Autodesk Inventor part; units mm, degrees
ref_plane "YZ Plane" through (0, 0, 0) normal (1, 0, 0) x (0, 1, 0)
ref_plane "XZ Plane" through (0, 0, 0) normal (0, 1, 0) x (-1, 0, 0)
ref_plane "XY Plane" through (0, 0, 0) normal (0, 0, 1) x (1, 0, 0)
sketch "Sketch1" plane through (0, 0, 0) normal (0, 0, 1) x (1, 0, 0)
  line L0 (0, 0) -> (-5, 0)
  line L1 (-5, 5) -> (-5, 50)
  line L2 (-5, 50) -> (0, 50)
  line L3 (0, 50) -> (0, 0)
  line L4 (0, 0) -> (-50, 0)
  line L5 (-50, 0) -> (-50, 5)
  line L6 (-50, 5) -> (-5, 5)
  line L7 (0, 5) -> (0, 0)
  dimension "d0" = 5
  dimension "d1" = 50
  dimension "d2" = 50
  dimension "d3" = 5
extrude "Extrusion1" add sketch "Sketch1" along normal blind 50
sketch "Sketch3" plane through (-50, 5, 0) normal (0, 1, 0) x (1, 0, 0)
  circle A0 centre (22.5, -25) radius 14.5
  line L0 (45, 0) -> (0, 0)
  line L1 (0, 0) -> (0, -50)
  line L2 (45, -50) -> (0, -50)
  line L3 (45, 0) -> (45, -50)
  line L4 (22.5, -25) -> (0, -25)
  line L5 (22.5, -25) -> (22.5, 0)
  line L6 (45, 0) -> (0, 0)
  circle A1 centre (35.935, -38.435) radius 2.75
  circle A2 centre (9.065, -38.435) radius 2.75
  circle A3 centre (22.5, -44) radius 2.75
  circle A4 centre (35.935, -11.565) radius 2.75
  circle A5 centre (9.065, -11.565) radius 2.75
  circle A6 centre (22.5, -6) radius 2.75
  point P0 (50, 0)
  dimension "d44" = 29
  dimension "d45" = 45
  dimension "d46" = 22.5
  dimension "d47" = 25
  dimension "d48" = 5.5
  dimension "d49" = 13.435
  dimension "d50" = 13.435
  dimension "d51" = 5.5
  dimension "d52" = 13.435
  dimension "d53" = 13.435
  dimension "d54" = 5.5
  dimension "d55" = 19
  dimension "d56" = 0
extrude "Extrusion2" cut sketch "Sketch3" against normal blind 20 contours A0 L4 L5 | L5 L4 A0 | A6 L5 | L5 A6 | A1 | A2 | A3 | A4 | A5
sketch "Sketch4" plane through (-5, 5, 0) normal (-1, 0, 0) x (0, 0, 1)
  circle A0 centre (17.5, 30) radius 2.75
  line L0 (0, 45) -> (0, 0)
  line L1 (0, 45) -> (50, 45)
  circle A1 centre (32.5, 30) radius 2.75
  point P0 (0, -5)
  dimension "d59" = 5.5
  dimension "d61" = 17.5
  dimension "d64" = 45
  dimension "d65" = 15
  dimension "d68" = 5.5
  dimension "d69" = 15
  dimension "d70" = 15
  dimension "d71" = 50
extrude "Extrusion3" cut sketch "Sketch4" against normal blind 20
equation "\"d2\" = d1"
equation "\"d3\" = d0"
equation "\"d46\" = 0.5 * d45"
equation "\"d50\" = d49"
equation "\"d52\" = d49"
equation "\"d53\" = d52"
equation "\"d61\" = -0.5 * d69 + 0.5 * d71"
equation "\"d65\" = -0.5 * d63 + 0.5 * d64"
equation "\"d70\" = d65"
properties part number "LBent_PScrew"
Check sheet for the modelled part. Datum: model origin and axes. Units: mm. A direction names the side the tool comes from. Round coordinates to 2 decimals unless told otherwise and drop trailing zeros. Order: outer loops, then holes, each group sorted by start corner. A loop starts at its lowest first (then second) coordinate and runs counter-clockwise, first axis right, second up.
Q1. Draft check along X on faces 3 (the face through (-13.67, 2.54, 20.64)), 4 (the face through (-38, 5, 36)), 5 (the face through (-29.527, 2.535, 42.141)), 6 (the face through (-50, 2, 25)). Enter one of: pulls with the +X half, pulls with the -X half, needs draft (parallel to the pull), parting line crosses it, or undercut.
Filled sheet:
face 3: undercut
face 4: needs draft
face 5: undercut
face 6: pulls with the -X half
Q2. Cross-section at A-A, the plane y = 35. Enter the section's corners in (x, z), plus the area to 3 significant figures.
Filled sheet:
outline: (-5, 0) - (0, 0) - (0, 14.75) - (-5, 14.75) - close; (-5, 20.25) - (0, 20.25) - (0, 29.75) - (-5, 29.75) - close; (-5, 35.25) - (0, 35.25) - (0, 50) - (-5, 50) - close
area: 195 mm2
Q3. Set-up check for faces 1 (the face through (-13.5, 0, 30.2)), 2 (the face through (-5, 27, 25)): record each of +Z, -Z, +X, -X, +Y, -Y from which the full face is reachable in a straight line by a thin tool's end or side.
Filled sheet:
face 1: +Z, -Z, +X, -X, -Y
face 2: +Z, -Z, -X, +Y
Q4. Scan lines: L1, parallel to Z at x = -27.5, y = 2.6; L2, parallel to Y at x = -23.5, z = 7; L3, parallel to X at y = 6.5, z = 32.5. Record each from-to range of solid material in increasing order.
Filled sheet:
L1: z = 0 to 3.25, 8.75 to 10.5, 39.5 to 41.25, 46.75 to 50
L2: y = 0 to 5
L3: x = -5 to 0
Q5. Cross-section at D-D, the plane z = 31. Enter the section's corners in (x, y), plus the area to 3 significant figures.
Filled sheet:
outline: (-50, 0) - (-40.7, 0) - (-40.7, 5) - (-50, 5) - close; (-14.3, 0) - (0, 0) - (0, 32.7) - (-5, 32.7) - (-5, 5) - (-14.3, 5) - close; (-5, 37.3) - (0, 37.3) - (0, 50) - (-5, 50) - close
area: 320 mm2
Q6. Cross-section at B-B, the plane z = 25. Enter the section's corners in (x, y).
Filled sheet:
outline: (-50, 0) - (-42, 0) - (-42, 5) - (-50, 5) - close; (-13, 0) - (0, 0) - (0, 50) - (-5, 50) - (-5, 5) - (-13, 5) - close
Q7. Cross-section at C-C, the plane x = -27.5. Enter the section's corners in (y, z).
Filled sheet:
outline: (0, 0) - (5, 0) - (5, 3.25) - (0, 3.25) - close; (0, 8.75) - (5, 8.75) - (5, 10.5) - (0, 10.5) - close; (0, 39.5) - (5, 39.5) - (5, 41.25) - (0, 41.25) - close; (0, 46.75) - (5, 46.75) - (5, 50) - (0, 50) - close
Q8. Depth check by flat-ended pin: P1, Ø9, axis at x = -40.935, z = 11.565, coming from the +Y side; P2, Ø2, axis at y = 21.5, z = 41, coming from the -X side. Enter the tip coordinate at first touch or a pass-through.
Filled sheet:
P1: stops at y = 5
P2: stops at x = -5
